from build123d import *

# Parameters (mm, degrees)
CROQUIS1_R              = 22.225
SALIENTE_EXTRUIR1_DEPTH = 31.75
CROQUIS2_R              = 4.445
CORTAR_EXTRUIR1_DEPTH   = 32.75
VACIADO1_T              = -6.35


with BuildPart() as part:
    # Croquis1 → Saliente-Extruir1 (new body)
    with BuildSketch(Plane(origin=(0, 0, 0), x_dir=(1, 0, 0), z_dir=(0, 1, 0))):
        Circle(CROQUIS1_R)
    extrude(amount=SALIENTE_EXTRUIR1_DEPTH)

    # Croquis2 → Cortar-Extruir1 (cut, through all)
    with BuildSketch(Plane(origin=(0, 31.75, 0), x_dir=(1, 0, 0), z_dir=(0, 1, 0))):
        with Locations((0, 22.225)):
            Circle(CROQUIS2_R)
        with Locations((19.247414599, -11.1125)):
            Circle(CROQUIS2_R)
        with Locations((-19.247414599, -11.1125)):
            Circle(CROQUIS2_R)
    extrude(amount=-CORTAR_EXTRUIR1_DEPTH, mode=Mode.SUBTRACT)

    # Vaciado1
    vaciado1_openings = [part.faces().sort_by_distance(p)[0] for p in [
        (0, 0, 0),
    ]]
    offset(amount=VACIADO1_T, openings=vaciado1_openings, kind=Kind.INTERSECTION)


solid = part.part
Design review of the part built by this model. Coordinates are the model's own, in mm. A direction names the side the tool comes from. Round coordinates to 2 decimals unless told otherwise and drop trailing zeros. Loops run counter-clockwise (first coordinate to the right, second up) from the corner with the lowest first, then second, coordinate; pieces in that order, holes last. Notation, with made-up numbers: (-37.75, 39.5) -> (-5.75, 39.5) arc R19 ccw to (-5.75, 55.5) -> close; hole circle Ø7 at (-1, 29.5). An arc over 180 degrees is marked (long way). Use one line per item in the form item = value. Start each with the question number.
Q1. Wall thickness on line 1 along Y through (x, z) = (6, 14.5); line 2 along X through (y, z) = (16.5, -7.5); line 3 along X through (y, z) = (4.5, -11): over which ranges is each line inside the solid? List them lowest first. Write a range as [from, to].
Q2. We need section C-C on z = -0.5. Give the boundary of the cut face in (x, y).
Q3. For pin 1 Ø5 at (x, y) = (-10.5, 5) entering from +Z; pin 2 Ø2 at (y, z) = (26, -1.5) entering from -X; pin 3 Ø1 at (y, z) = (17, -2) entering from +X; pin 4 Ø2 at (x, z) = (7.5, -14.5) entering from -Y, all flat-tipped, find the tip position at first contact; note any pin that passes through.
Q4. We need section D-D on x = -3. Give the boundary of the cut face in (y, z).
Q5. Machinability: for faces 1 (the face through (-0.128, 12.522, 15.874)), 2 (the face through (-19.114, 15.653, -11.34)), which of the approach directions +Z, -Z, +X, -X, +Y, -Y give a long, thin tool a straight path to every point of the face, cutting with its end or side? Answer none if there is none.
Q6. Draft analysis for pull direction Z (two halves, no side actions). For faces 3 (the face through (10, 0, 10)), 4 (the face through (-0.09, 16.1, -17.78)), 5 (the face through (15.445, 16.097, 8.811)), 6 (the face through (-0.263, 15.653, 22.223)), state which applies: +Z half, -Z half, draft (parallel to the pull), parting line (faces both ways), or undercut.
Calculated:
q1.line_1 = [25.4, 31.75]
q1.line_2 = [-20.92, -13.99], [13.99, 20.92]
q1.line_3 = [-19.31, -11.45], [11.45, 19.31]
q2.outline = (-22.22, 0) -> (-15.87, 0) -> (-15.87, 25.4) -> (15.87, 25.4) -> (15.87, 0) -> (22.22, 0) -> (22.22, 31.75) -> (-22.22, 31.75) -> close
q3.pin_1 = 20.74
q3.pin_2 = -22.22
q3.pin_3 = 22.17
q3.pin_4 = 0
q4.outline = (0, -18.95) -> (31.75, -18.95) -> (31.75, 22.02) -> (0, 22.02) -> (0, 15.59) -> (25.4, 15.59) -> (25.4, -11.86) -> (0, -11.86) -> close
q5.face_1 = -Y
q5.face_2 = -X, +Y, -Y
q6.face_3 = draft
q6.face_4 = -Z half
q6.face_5 = undercut
q6.face_6 = +Z half
